Here's how the part is built. I have some questions about the finished solid (model axes, mm). Coordinates: 2 decimals unless noted, no trailing zeros. Order: outer loops, then holes, each group sorted by start corner. A loop starts at its lowest first (then second) coordinate and runs counter-clockwise, first axis right, second up. Notation, with made-up numbers: (37.25, -2) - (89.25, -2) arc R16 ccw to (89.25, 2) - close; hole circle Ø7 at (-19, 15.5). An arc over 180 degrees is marked (long way). Answer in a Markdown table with one row per item. Add a question column.
Item 1: I want a section at A-A (x = 150). Please give me the cut outline in (y, z), plus the area to 3 significant figures.
Item 2: Thinking about a two-plate mould opening in Z: for faces 1 (the flat face through (546, 76, 645)), 2 (the cylindrical face through (95.236, 73.95, 566.421)), 3 (the flat face through (135, 74, 385.259)), 4 (the flat face through (273.936, 74, 190)), which applies, +Z half, -Z half, draft (parallel to the pull), parting line (faces both ways), or undercut?
Item 3: I want a section at D-D (y = 24). Please give me the cut outline in (x, z), plus the area to 3 significant figures.
Item 4: I want a section at C-C (y = 75). Please give me the cut outline in (x, z), plus the area to 3 significant figures.
Item 5: If I drill on line 1 along Y through (x, z) = (1048, 509); line 2 along X through (y, z) = (50, 495); line 3 along X through (y, z) = (117, 495), over which ranges is the centre line in solid material (lowest first)? Write a range as from..to.
Item 6: I want a section at B-B (z = 495). Please give me the cut outline in (x, y), plus the area to 3 significant figures.
Item 7: Will these pins go through, and if not, where does the flat tip stop? pin 1 Ø6 at (y, z) = (119.5, 264.5) entering from -X; pin 2 Ø3 at (x, y) = (161, 109) entering from -Z; pin 3 Ø1.5 at (y, z) = (32, 176) entering from +X.
```python
from build123d import *

# Parameters (mm, degrees)
SKETCH1_W           = 1106.97250468
SKETCH1_H           = 150
BOSS_EXTRUDE1_DEPTH = 645
SKETCH2_R           = 90
CUT_EXTRUDE1_DEPTH  = 1290.927566229
SKETCH3_W           = 273.936328983
SKETCH3_H           = 385.258703225
CUT_EXTRUDE2_DEPTH  = 1290.927566229
CUT_EXTRUDE3_DEPTH  = 1290.927566229


with BuildPart() as part:
    # Sketch1 → Boss-Extrude1 (new body)
    with BuildSketch(Plane.XY):
        with Locations((553.48625234, 75)):
            Rectangle(SKETCH1_W, SKETCH1_H)
    extrude(amount=BOSS_EXTRUDE1_DEPTH)

    # Sketch2 → Cut-Extrude1 (cut, through all)
    with BuildSketch(Plane.XZ):
        with Locations(Location((150, 495, 0), (0, 0, 270))):
            Circle(SKETCH2_R)
    extrude(amount=-CUT_EXTRUDE1_DEPTH, mode=Mode.SUBTRACT)

    # Sketch3 → Cut-Extrude2 (cut, through all)
    with BuildSketch(Plane.XZ):
        with Locations((136.968164492, 192.629351613)):
            Rectangle(SKETCH3_W, SKETCH3_H)
    extrude(amount=-CUT_EXTRUDE2_DEPTH, mode=Mode.SUBTRACT)

    # Sketch5 → Cut-Extrude3 (cut, through all)
    with BuildSketch(Plane.XY.offset(645)):
        with BuildLine():
            Line((1106.97250468, 150), (1106.97250468, 0))
            ThreePointArc((1106.97250468, 0), (1031.97250468, 75), (1106.97250468, 150))
        make_face()
    extrude(amount=-CUT_EXTRUDE3_DEPTH, mode=Mode.SUBTRACT)


solid = part.part
```
Values follow:
| question | item | result |
|---|---|---|
| 1 | outline | (0, 385.26) - (150, 385.26) - (150, 405) - (0, 405) - close; (0, 585) - (150, 585) - (150, 645) - (0, 645) - close |
| 1 | area | 12,000 mm^2 |
| 2 | face 1 | +Z half |
| 2 | face 2 | undercut |
| 2 | face 3 | -Z half |
| 2 | face 4 | draft |
| 3 | outline | (0, 385.26) - (273.94, 385.26) - (273.94, 0) - (1051.98, 0) - (1051.98, 645) - (0, 645) - close; hole circle Ø180 at (150, 495) |
| 3 | area | 548,000 mm^2 |
| 4 | outline | (0, 385.26) - (273.94, 385.26) - (273.94, 0) - (1031.97, 0) - (1031.97, 645) - (0, 645) - close; hole circle Ø180 at (150, 495) |
| 4 | area | 535,000 mm^2 |
| 5 | line 1 | y = 0..28.66, 121.34..150 |
| 5 | line 2 | x = 0..60, 240..1036.26 |
| 5 | line 3 | x = 0..60, 240..1044.84 |
| 6 | outline | (0, 0) - (60, 0) - (60, 150) - (0, 150) - close; (240, 0) - (1106.97, 0) arc R75 cw to (1106.97, 150) - (240, 150) - close |
| 6 | area | 130,000 mm^2 |
| 7 | pin 1 | stops at x = 273.94 |
| 7 | pin 2 | stops at z = 385.26 |
| 7 | pin 3 | stops at x = 1046.06 |
